Could you check a few things on this model? Use its own coordinates, in mm. A direction names the side the tool comes from. Round coordinates to 2 decimals unless told otherwise and drop trailing zeros. Loops run counter-clockwise (first coordinate to the right, second up) from the corner with the lowest first, then second, coordinate; pieces in that order, holes last. Notation, with made-up numbers: M -0.75,25.25 L 54.25,25.25 A15 ccw 54.25,44.25 Z; hole C 53,17.25 d2. An arc over 180 degrees is marked long. Return JSON: item names as keys, results as strings. Group by question number.
```python
from build123d import *

# Parameters (mm, degrees)
F1_DEPTH     = 1
F2_W         = 1.7
F2_H         = 2
F2_W_2       = 6.3
F2_H_2       = 8
F3_DEPTH     = 1.7
F4_W         = 8
F4_H         = 10
F5_DEPTH     = 2
F6_R         = 5
F7_R         = 0.99999
F8_T1_DEPTH  = 3.7
F8_T3_DEPTH  = 7.5
F8_T5_DEPTH  = 9.5
F8_T7_DEPTH  = 5.5
F8_T9_DEPTH  = 11.5
F8_T12_ANGLE = 90
F8_S15_W     = 1
F8_S15_H     = 1
F8_T16_DEPTH = 1
F8_T20_ANGLE = 90
F10_DEPTH    = 1.7


# Not quite as in the source:
# - a fillet or chamfer that OpenCascade refuses, or shapes differently, is made with other operations: its cross-section is extruded or revolved along the edge and cut away or added
# - a fillet or chamfer is up to 0.001 mm smaller than in the source, because OpenCascade refuses the exact size


with BuildPart() as f1:
    # F0 (on Top) → F1 (new body)
    with BuildSketch(Plane.XY):
        with BuildLine():
            Line((-6.5, -51), (6.5, -51))
            Line((6.5, -51), (6.5, 46))
            ThreePointArc((6.5, 46), (5.0355339059, 49.5355339059), (1.5, 51))
            Line((1.5, 51), (-6.5, 51))
            Line((-6.5, 51), (-6.5, -51))
        make_face()
    extrude(amount=F1_DEPTH)

    # F2 (on face) → F3 (join)
    with BuildSketch(Plane(origin=(0, 0, 0), x_dir=(1, 0, 0), z_dir=(0, 0, -1))):
        with Locations((-5.65, -50)):
            Rectangle(F2_W, F2_H)
        with Locations((-1.65, -50)):
            Rectangle(F2_W_2, F2_H)
        with Locations((-5.65, -45)):
            Rectangle(F2_W, F2_H_2)
    extrude(amount=F3_DEPTH)

    # F4 (on face) → F5 (join)
    with BuildSketch(Plane(origin=(0, 0, -1.7), x_dir=(1, 0, 0), z_dir=(0, 0, -1))):
        with Locations((-2.5, -46)):
            Rectangle(F4_W, F4_H)
    extrude(amount=F5_DEPTH)

    # F6
    f6_edges = [f1.edges().sort_by_distance(p)[0] for p in [
        (6.5, -51, 0.5),
        (1.5, 41, -2.7),
    ]]
    fillet(f6_edges, radius=F6_R)

    # F7 (radius 1 in the source; OpenCascade refuses exactly that, so slightly less here)
    f7_edges = [f1.edges().sort_by_distance(p)[0] for p in [
        (-2.5, -51, 1),
        (5.035534, -49.535534, 1),
        (-6.5, 0, 1),
        (6.5, 0, 1),
        (-2.5, 51, 1),
        (5.035534, 49.535534, 1),
    ]]
    fillet(f7_edges, radius=F7_R)

    # F8: fillet of radius 1 on 6 edges, made by hand

    # F8_s2 → F8_t1 (cut)
    with BuildSketch(Plane.XY.offset(-2.7)):
        with BuildLine():
            ThreePointArc((-5.5, 51), (-6.2071067812, 50.7071067812), (-6.5, 50))
            Line((-6.5, 50), (-6.5, 51))
            Line((-6.5, 51), (-5.5, 51))
        make_face()
    extrude(amount=F8_T1_DEPTH, mode=Mode.SUBTRACT)

    # F8_s4 → F8_t3 (cut)
    with BuildSketch(Plane.XZ.offset(-53.5)):
        with BuildLine():
            ThreePointArc((1.5, -2.7), (1.2071067812, -3.4071067812), (0.5, -3.7))
            Line((0.5, -3.7), (1.5, -3.7))
            Line((1.5, -3.7), (1.5, -2.7))
        make_face()
    extrude(amount=F8_T3_DEPTH, mode=Mode.SUBTRACT)

    # F8_s6 → F8_t5 (cut)
    with BuildSketch(Plane.YZ.offset(-5.5)):
        with BuildLine():
            ThreePointArc((51, -2.7), (50.7071067812, -3.4071067812), (50, -3.7))
            Line((50, -3.7), (51, -3.7))
            Line((51, -3.7), (51, -2.7))
        make_face()
    extrude(amount=F8_T5_DEPTH, mode=Mode.SUBTRACT)

    # F8_s8 → F8_t7 (cut)
    with BuildSketch(Plane.YZ.offset(-9)):
        with BuildLine():
            ThreePointArc((42, -3.7), (41.2928932188, -3.4071067812), (41, -2.7))
            Line((41, -2.7), (41, -3.7))
            Line((41, -3.7), (42, -3.7))
        make_face()
    extrude(amount=F8_T7_DEPTH, mode=Mode.SUBTRACT)

    # F8_s10 → F8_t9 (cut)
    with BuildSketch(Plane.XZ.offset(-50)):
        with BuildLine():
            ThreePointArc((-6.5, -2.7), (-6.2071067812, -3.4071067812), (-5.5, -3.7))
            Line((-5.5, -3.7), (-6.5, -3.7))
            Line((-6.5, -3.7), (-6.5, -2.7))
        make_face()
    extrude(amount=F8_T9_DEPTH, mode=Mode.SUBTRACT)

    # F8_s11 → F8_t12 (revolve, cut)
    with BuildSketch(Plane.YZ.offset(-5.5)):
        with BuildLine():
            ThreePointArc((50.00001, 1), (50.7071097101, 0.7071097101), (51, 1e-05))
            Line((51, 1e-05), (51, 1))
            Line((51, 1), (50.00001, 1))
        make_face()
    revolve(axis=Axis((-5.5, 50, 1), (0, 0, 1)), revolution_arc=F8_T12_ANGLE, mode=Mode.SUBTRACT)


with BuildPart() as f8_tool14:
    # F8_s15 → F8_t16 (new body)
    with BuildSketch(Plane.XZ.offset(-50)):
        with Locations((-6, -3.2)):
            Rectangle(F8_S15_W, F8_S15_H)
    extrude(amount=-F8_T16_DEPTH)

    # F8_s17 → F8_t18 (revolve, cut)
    with BuildSketch(Plane(origin=(-5.5, 50, -2.7), x_dir=(0.7071067812, 0, 0.7071067812), z_dir=(-0.7071067812, 0, 0.7071067812))):
        with BuildLine():
            ThreePointArc((0, -1), (1, 0), (0, 1))
            Line((0, 1), (0, -1))
        make_face()
    revolve(axis=Axis((-5.5, 50, -2.7), (0, 1, 0)), mode=Mode.SUBTRACT)


with BuildPart() as f1_1:
    add(f1.part)

    # F8_t13: cut F8_tool14
    add(f8_tool14.part, mode=Mode.SUBTRACT)

    # F8_s19 → F8_t20 (revolve, cut)
    with BuildSketch(Plane.XZ.offset(-46)):
        with BuildLine():
            ThreePointArc((0.5, -3.7), (1.2071067812, -3.4071067812), (1.5, -2.7))
            Line((1.5, -2.7), (1.5, -3.7))
            Line((1.5, -3.7), (0.5, -3.7))
        make_face()
    revolve(axis=Axis((-3.5, 46, -3.7), (0, 0, -1)), revolution_arc=F8_T20_ANGLE, mode=Mode.SUBTRACT)

    # F9 (on face) → F10 (join, through all)
    with BuildSketch(Plane(origin=(0, 0, 0), x_dir=(1, 0, 0), z_dir=(0, 0, -1))):
        with BuildLine():
            ThreePointArc((-3.5, -42), (-0.6715728753, -43.1715728753), (0.5, -46))
            Line((0.5, -46), (1.5, -46))
            ThreePointArc((1.5, -46), (0.0355339059, -42.4644660941), (-3.5, -41))
            Line((-3.5, -41), (-3.5, -42))
        make_face()
    extrude(amount=F10_DEPTH)


solid = f1_1.part
```
1. I'm going to push flat-ended pins straight in: pin 1 Ø0.8 at (y, z) = (47.5, -1) entering from +X; pin 2 Ø3 at (x, y) = (5, 7) entering from -Z; pin 3 Ø1.9 at (x, z) = (-0.5, -1) entering from -Y. Where does each tip first touch, or does it pass through?
2. We'd pull the mould along X, two halves only. Please class faces 1 (the face through (-4.8, 45, -1)), 2 (the face through (-6.5, 48, -1)), 3 (the face through (1.5, 49, -2)): +X half, -X half, draft (parallel to the pull), parting line (faces both ways), or undercut.
3. I need wall thicknesses on probe 1 along Z at (x, y) = (-4.25, -45); probe 2 along Y at (x, z) = (-4.25, 0.2); probe 3 along X at (y, z) = (27.5, 0.2). Which ranges of each line are inside material? Lowest first, please.
4. If we section it at A-A, the plane z = -0.9: Please give me the cut outline in (x, y).
5. On a 3-axis mill with a long thin cutter (end or side, diameter ignored), from which of +Z, -Z, +X, -X, +Y, -Y can I reach the whole of each face in a straight line? I mean faces 4 (the face through (-2, 46, -1.7)), 5 (the face through (-2, 49, -1)), 6 (the face through (-5, 41, -2)), 7 (the face through (0, 1, 1)). Say none if no direction works.
Geometry results:
{
 "1": {"pin 1": "x = -4.8", "pin 2": "z = 0", "pin 3": "y = 41.44"},
 "2": {"face 1": "undercut", "face 2": "-X half", "face 3": "+X half"},
 "3": {"probe 1": "0 to 1", "probe 2": "-50.98 to 50.98", "probe 3": "-6.48 to 6.48"},
 "4": {"outline": "M -6.5,41 L -4.8,41 L -4.8,49 L 1.5,49 L 1.5,51 L -5.5,51 A1 ccw -6.5,50 Z; M -3.5,41 A5 ccw 1.5,46 L 0.5,46 A4 cw -3.5,42 Z"},
 "5": {"face 4": "none", "face 5": "+X", "face 6": "-Z, +X, -X, -Y", "face 7": "+Z, +X, -X, +Y, -Y"}
}
